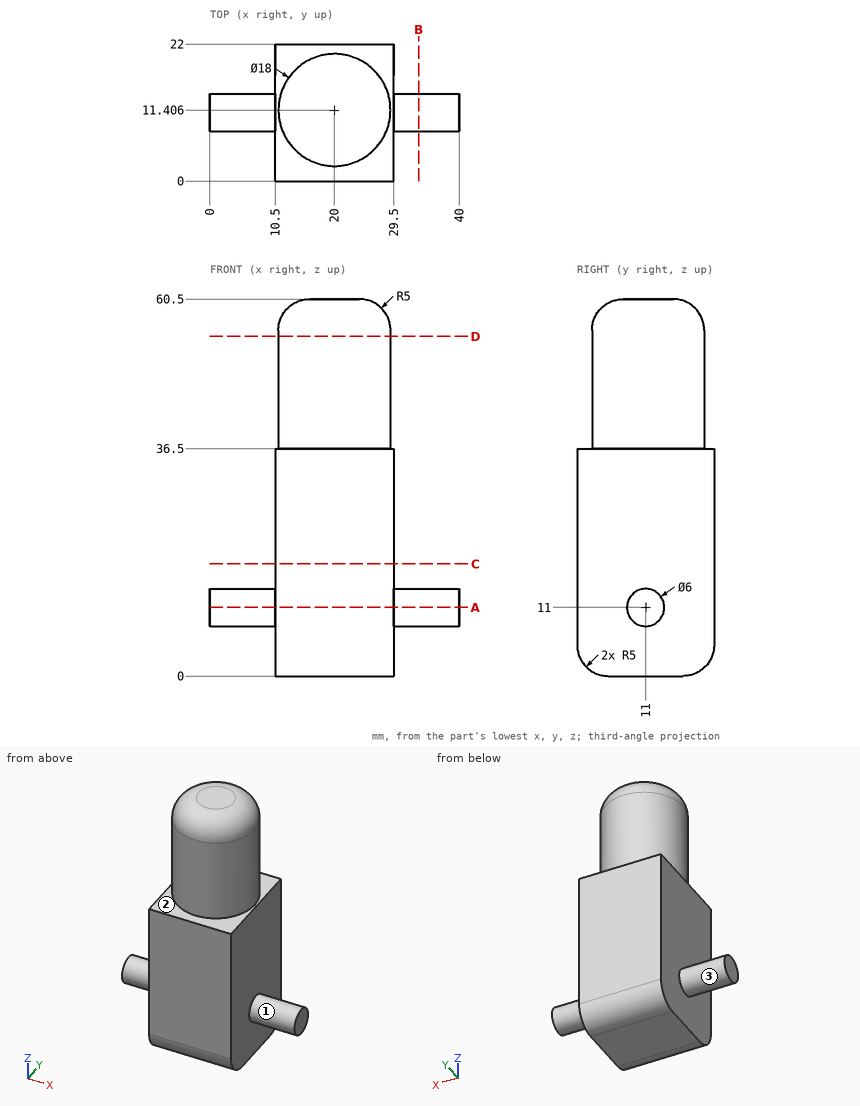
Geometry check sheet. Reference: drawing and pictorial views, mm from the part's lowest x, y, z. A direction names the side the tool comes from. Give positions to 0.01 mm unless a question says otherwise; leave off trailing zeros. Order: outer loops, then holes, each group sorted by start corner. A loop starts at its lowest first (then second) coordinate and runs counter-clockwise, first axis right, second up. Notation, with made-up numbers: M 73,-2.75 L 106,-2.75 A15 ccw 106,26.25 Z; hole C -15,79 d2. An arc over 180 degrees is marked long. Answer in a Markdown table with one row per item. Add a question column.
Q1. Sectioned sample at A-A, the plane z = 11. Record the boundary of the cut face in (x, y), and give its area (3 significant figures).
Q2. Thickness scan on L1, parallel to X at y = 7.5, z = 35.5; L2, parallel to Z at x = 28, y = 6.75; L3, parallel to X at y = 18.5, z = 44 (1 decimal). Record the ranges inside material, lowest first.
Q3. Sectioned sample at C-C, the plane z = 18. Record the boundary of the cut face in (x, y), and give its area (3 significant figures).
Q4. Sectioned sample at D-D, the plane z = 54.5. Record the boundary of the cut face in (x, y) (1 decimal).
Q5. Access from +Z, -Z, +X, -X, +Y, -Y to the whole of each face (thin tool, end or side, straight path). Record for the marked faces 1, 2 and 3.
Q6. Gauge pin test, flat ends, axial feed: pin 1 Ø6 at (y, z) = (15.5, 20.5) entering from +X; pin 2 Ø12 at (x, y) = (6, 18) entering from +Z; pin 3 Ø5 at (y, z) = (9.5, 48) entering from +X; pin 4 Ø1.5 at (x, y) = (34, 6.5) entering from -Z. Record the tip position at first contact, or that the pin passes through.
Q7. Sectioned sample at B-B, the plane x = 33.5. Record the boundary of the cut face in (y, z).
Verdict:
| question | item | result |
|---|---|---|
| 1 | outline | M 0,8 L 10.5,8 L 10.5,0 L 29.5,0 L 29.5,8 L 40,8 L 40,14 L 29.5,14 L 29.5,22 L 10.5,22 L 10.5,14 L 0,14 Z |
| 1 | area | 544 mm² |
| 2 | L1 | 10.5 to 29.5 |
| 2 | L2 | 0 to 36.5 |
| 2 | L3 | 14.5 to 25.5 |
| 3 | outline | M 10.5,0 L 29.5,0 L 29.5,22 L 10.5,22 Z |
| 3 | area | 418 mm² |
| 4 | outline | C 20,11.4 d18 |
| 5 | face 1 | +X |
| 5 | face 2 | +Z |
| 5 | face 3 | -X |
| 6 | pin 1 | x = 29.5 |
| 6 | pin 2 | z = 36.5 |
| 6 | pin 3 | x = 29 |
| 6 | pin 4 | through |
| 7 | outline | C 11,11 d6 |
